from build123d import *

# Parameters (mm, degrees)
ESQUISSE1_R             = 8
BOSS_EXTRU_1_DEPTH      = 15
BOSS_EXTRU_1_TAPER      = 5
ESQUISSE2_R             = 2.5
ENL_V_MAT_EXTRU_1_DEPTH = 30
ESQUISSE3_R             = 4
ENL_V_MAT_EXTRU_2_DEPTH = 10
CONG_2_R                = 0.5
CONG_3_R                = 0.5
CONG_4_R                = 0.5


with BuildPart() as part:
    # Esquisse1 → Boss.-Extru.1 (new body)
    with BuildSketch(Plane.XY):
        Circle(ESQUISSE1_R)
    extrude(amount=BOSS_EXTRU_1_DEPTH, taper=BOSS_EXTRU_1_TAPER)

    # Esquisse2 → Enlèv. mat.-Extru.1 (cut)
    with BuildSketch(Plane.XY.offset(15)):
        Circle(ESQUISSE2_R)
    extrude(amount=-ENL_V_MAT_EXTRU_1_DEPTH, mode=Mode.SUBTRACT)

    # Esquisse3 → Enlèv. mat.-Extru.2 (cut)
    with BuildSketch(Plane.XY.offset(15)):
        Circle(ESQUISSE3_R)
    extrude(amount=-ENL_V_MAT_EXTRU_2_DEPTH, mode=Mode.SUBTRACT)

    # Congé2
    cong_2_edges = [part.edges().sort_by_distance(p)[0] for p in [
        (-4, 0, 15),
    ]]
    fillet(cong_2_edges, radius=CONG_2_R)

    # Congé3
    cong_3_edges = [part.edges().sort_by_distance(p)[0] for p in [
        (-8, 0, 0),
    ]]
    fillet(cong_3_edges, radius=CONG_3_R)

    # Congé4
    cong_4_edges = [part.edges().sort_by_distance(p)[0] for p in [
        (-6.687670047, 0, 15),
    ]]
    fillet(cong_4_edges, radius=CONG_4_R)


solid = part.part
Model file for the job. Use its own axes, mm. A direction names the side the tool comes from. Coordinates: 2 decimals unless noted, no trailing zeros. Write each loop counter-clockwise with the first axis right and the second up, starting at its lowest first coordinate (ties: lowest second). Pieces come first, ordered by that corner, then holes. Notation, with made-up numbers: (44.5, 62) - (73.5, 62) arc R8 cw to (73.5, 75) - close; hole circle Ø10 at (-18.75, 58). An arc over 180 degrees is marked (long way). Write each question's results on one line, items separated by ' | '. Start each with the question number.
1) Mould opens along Y. For faces 3 (the face through (2, 2, 5)), 4 (the face through (-0.95, 7.27, 7.64)), 5 (the face through (4, -3, 15)) say: pulls with the +Y half, pulls with the -Y half, needs draft (parallel to the pull), parting line crosses it, or undercut.
2) Cut at A-A (y = 0). Write the cut outline in (x, z).
3) 3-axis set-ups, long thin cutter, end or side, ignore diameter. For faces 1 (the face through (-0.867, -3.905, 9.817)), 2 (the face through (-0.54, -2.44, 2.54)): which of +Z, -Z, +X, -X, +Y, -Y reach the whole face in a straight line?
4) Cut at D-D (z = 13.25). Write the cut outline in (x, y), then the cut area to 3 significant figures.
5) Flat gauge pins, fed straight in: P1, Ø1, axis at x = 2.5, z = 5, coming from the +Y side; P2, Ø2.5, axis at x = -1, y = 1, coming from the +Z side; P3, Ø1.5, axis at y = -1, z = 6.5, coming from the +X side. Where does each tip first touch, or does it go through?
6) Probe line 1 along Z through (x, y) = (-0.5, -3.5); line 2 along X through (y, z) = (2, 9.5); line 3 along X through (y, z) = (2.25, 11.5). List the from-to ranges inside material, lowest first. Write a range as from..to.
7) Cut at C-C (z = 4). Write the cut outline in (x, y), then the cut area to 3 significant figures.
Returned:
1) face 3: undercut | face 4: parting line crosses it | face 5: needs draft
2) outline: (-7.95, 0.54) arc R0.5 ccw to (-7.45, 0) - (-2.5, 0) - (-2.5, 5) - (-4, 5) - (-4, 14.5) arc R0.5 ccw to (-4.5, 15) - (-6.23, 15) arc R0.5 ccw to (-6.73, 14.54) - close; (2.5, 0) - (7.45, 0) arc R0.5 ccw to (7.95, 0.54) - (6.73, 14.54) arc R0.5 ccw to (6.23, 15) - (4.5, 15) arc R0.5 ccw to (4, 14.5) - (4, 5) - (2.5, 5) - close
3) face 1: +Z | face 2: +Z, -Z
4) outline: circle Ø13.68 at (0, 0); hole circle Ø8 at (0, 0) | area: 96.7 mm^2
5) P1: y = 7.3 | P2: z = 5 | P3: x = 7.46
6) line 1: 0..5 | line 2: -6.88..-3.46, 3.46..6.88 | line 3: -6.62..-3.31, 3.31..6.62
7) outline: circle Ø15.3 at (0, 0); hole circle Ø5 at (0, 0) | area: 164 mm^2
